from build123d import *

# Parameters (mm, degrees)
SKETCH_1_R          = 1.5
SKETCH_1_R_2        = 11
SKETCH_1_R_3        = 3
EXTRUDE_1_DEPTH     = 4
CUT_EXTRUDE_1_DEPTH = 10


with BuildPart() as part:
    # 草图1 → 凸台-拉伸1 (new body)
    with BuildSketch(Plane(origin=(0, 0, 0), x_dir=(0, 0, -1), z_dir=(1, 0, 0))):
        with BuildLine():
            Line((-61.155133648, -62), (-61.155133648, -70))
            Line((-61.155133648, -70), (12, -70))
            Line((12, -70), (12, -62))
            Line((12, -62), (12, 0))
            ThreePointArc((12, 0), (10.643645992, 5.541913027), (6.8812, 9.83102673))
            ThreePointArc((6.8812, 9.83102673), (3.607469975, 11.44491854), (0, 12))
            Line((0, 12), (-61.155133648, 12))
            Line((-61.155133648, 12), (-61.155133648, -62))
        make_face()
        with Locations((-51.155133648, -62)):
            Circle(SKETCH_1_R, mode=Mode.SUBTRACT)
        with Locations((-41.155133648, -62)):
            Circle(SKETCH_1_R, mode=Mode.SUBTRACT)
        with Locations((-47.319805147, -47.319805147)):
            Circle(SKETCH_1_R, mode=Mode.SUBTRACT)
        with Locations((-31.819805153, -31.819805153)):
            Circle(SKETCH_1_R_2, mode=Mode.SUBTRACT)
        with Locations((-8, -62)):
            Circle(SKETCH_1_R, mode=Mode.SUBTRACT)
        with Locations((2, -62)):
            Circle(SKETCH_1_R, mode=Mode.SUBTRACT)
        with Locations((-16.319805153, -47.319805147)):
            Circle(SKETCH_1_R, mode=Mode.SUBTRACT)
        with Locations((-47.319805147, -16.319805153)):
            Circle(SKETCH_1_R, mode=Mode.SUBTRACT)
        with Locations((-16.319805153, -16.319805153)):
            Circle(SKETCH_1_R, mode=Mode.SUBTRACT)
        Circle(SKETCH_1_R_3, mode=Mode.SUBTRACT)
    extrude(amount=EXTRUDE_1_DEPTH)

    # 草图2 → 切除-拉伸1 (cut)
    with BuildSketch(Plane(origin=(4, 0, 0), x_dir=(0, 0, -1), z_dir=(1, 0, 0))):
        with BuildLine():
            Line((-55.384065837, 4.928932188), (-55.384065837, -0.071067812))
            ThreePointArc((-55.384065837, -0.071067812), (-54.084065837, -1.371067812), (-52.784065837, -0.071067812))
            Line((-52.784065837, -0.071067812), (-52.784065837, 4.928932188))
            ThreePointArc((-52.784065837, 4.928932188), (-54.084065837, 6.228932188), (-55.384065837, 4.928932188))
        make_face()
        with BuildLine():
            Line((-45.884065837, 4.928932188), (-45.884065837, -0.071067812))
            ThreePointArc((-45.884065837, -0.071067812), (-44.584065837, -1.371067812), (-43.284065837, -0.071067812))
            Line((-43.284065837, -0.071067812), (-43.284065837, 4.928932188))
            ThreePointArc((-43.284065837, 4.928932188), (-44.584065837, 6.228932188), (-45.884065837, 4.928932188))
        make_face()
    extrude(amount=-CUT_EXTRUDE_1_DEPTH, mode=Mode.SUBTRACT)


solid = part.part
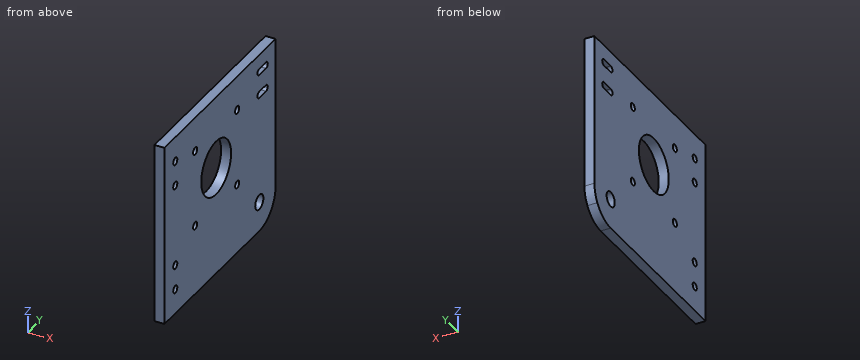
For this review, take the finished solid that the model builds, in its own axes (mm). Round coordinates to 2 decimals unless told otherwise and drop trailing zeros. Loops run counter-clockwise (first coordinate to the right, second up) from the corner with the lowest first, then second, coordinate; pieces in that order, holes last. Notation, with made-up numbers: (5.5, 82.5) - (10.5, 82.5) arc R25 cw to (10.5, 118.5) - close; hole circle Ø8 at (78.25, -14.75). An arc over 180 degrees is marked (long way). Use one line per item in the form item = value.
1) We need section C-C on y = -26.5. Write out the cut boundary in (x, z).
Solutions:
outline = (0, -12) - (4, -12) - (4, 22.19) - (0, 22.19) - close; (0, 41.45) - (4, 41.45) - (4, 61.16) - (0, 61.16) - close
2) We need section D-D on x = 0.65. State how many separate pieces and enclosed holes the cut face has, then the cut area to 3 significant figures.
Solutions:
separate_pieces = 1
enclosed_holes = 12
area = 5,470 mm2
3) Wall thickness on probe 1 along Z at (x, y) = (2.1, -48); probe 2 along Z at (x, y) = (0.4, -47); probe 3 along Y at (x, z) = (0.35, 8): over which ranges is each line inside the solid? List them lowest first.
Solutions:
probe_1 = -12 to 14.98, 17.66 to 45.98, 48.66 to 61.16
probe_2 = -12 to 14.85, 17.79 to 45.85, 48.79 to 61.16
probe_3 = -70 to -63.5, -60.5 to 12
4) We need section B-B on y = -62. Write out the cut boundary in (x, z), then the cut area to 3 significant figures.
Solutions:
outline = (0, -12) - (4, -12) - (4, -3.5) - (0, -3.5) - close; (0, -0.5) - (4, -0.5) - (4, 6.5) - (0, 6.5) - close; (0, 9.5) - (4, 9.5) - (4, 39.66) - (0, 39.66) - close; (0, 42.66) - (4, 42.66) - (4, 49.66) - (0, 49.66) - close; (0, 52.66) - (4, 52.66) - (4, 61.16) - (0, 61.16) - close
area = 245 mm2
5) We need section A-A on z = 8. Write out the cut boundary in (x, y).
Solutions:
outline = (0, -70) - (4, -70) - (4, -63.5) - (0, -63.5) - close; (0, -60.5) - (4, -60.5) - (4, 12) - (0, 12) - close
